```python
from build123d import *

# Parameters (mm, degrees)
SKETCH010_R             = 4
SKETCH010_R_2           = 1.5
PAD_DEPTH               = 10
POCKET003_DEPTH         = 5
POCKET004_DEPTH         = 2.7
PAD010_DEPTH            = 20
FILLET001_R             = 9
FILLET002_R             = 3
FILLET003_R             = 3
FILLET004_R             = 0.9
CHAMFER_SIZE            = 2
FILLET005_R             = 0.9
FILLET006_R             = 1
FILLET007_R             = 0.5
FILLET008_R             = 0.3
FILLET009_R             = 1
BODY001_PLACEMENT_ANGLE = 45


with BuildPart() as part:
    # Sketch010 → Pad (new body)
    with BuildSketch(Plane.XY):
        Polygon((-45.961941, -24.748737), (0, 21.213203), (21.213203, 0), (-24.748737, -45.961941), align=None)
        with Locations((-7.071068, -7.071068)):
            Circle(SKETCH010_R, mode=Mode.SUBTRACT)
        with Locations((-7.071068, 7.071068)):
            Circle(SKETCH010_R_2, mode=Mode.SUBTRACT)
        with Locations((7.071068, -7.071068)):
            Circle(SKETCH010_R_2, mode=Mode.SUBTRACT)
    extrude(amount=PAD_DEPTH)

    # Sketch011 → Pocket003 (cut)
    with BuildSketch(Plane.XY.offset(10)):
        Polygon((-47.335856, -39.41626), (26.386553, 34.306149), (34.306149, 26.386553), (-39.41626, -47.335856), align=None)
    extrude(amount=-POCKET003_DEPTH, mode=Mode.SUBTRACT)

    # Sketch017 → Pocket004 (cut)
    with BuildSketch(Plane.XY.offset(10)):
        with BuildLine():
            ThreePointArc((-5.6, 10.6), (-9.135534, 9.135534), (-10.6, 5.6))
            Line((-10.6, 5.6), (-10.6, -5.6))
            ThreePointArc((-10.6, -5.6), (-9.135534, -9.135534), (-5.6, -10.6))
            Line((-5.6, -10.6), (5.6, -10.6))
            ThreePointArc((5.6, -10.6), (9.135534, -9.135534), (10.6, -5.6))
            Line((10.6, -5.6), (10.6, 5.6))
            ThreePointArc((10.6, 5.6), (9.135534, 9.135534), (5.6, 10.6))
            Line((5.6, 10.6), (-5.6, 10.6))
        make_face()
    extrude(amount=-POCKET004_DEPTH, mode=Mode.SUBTRACT)

    # Sketch023 → Pad010 (join)
    with BuildSketch(Plane.XY.offset(10)):
        Polygon((-41.7193, -21.92031), (-39.59798, -24.041631), (-43.133514, -27.577164), (-45.254834, -25.455844), align=None)
        Polygon((-24.960869, -5.16188), (-22.839549, -7.2832), (-19.304015, -3.747666), (-21.425335, -1.626346), align=None)
    extrude(amount=PAD010_DEPTH)

    # Fillet001
    fillet001_edges = [part.edges().sort_by_distance(p)[0] for p in [
        (0, 21.213203, 5),
        (21.213203, 0, 5),
    ]]
    fillet(fillet001_edges, radius=FILLET001_R)

    # Fillet002
    fillet002_edges = [part.edges().sort_by_distance(p)[0] for p in [
        (-45.961941, -24.748737, 5),
        (-24.748737, -45.961941, 5),
    ]]
    fillet(fillet002_edges, radius=FILLET002_R)

    # Fillet003
    fillet003_edges = [part.edges().sort_by_distance(p)[0] for p in [
        (-41.365747, -25.809398, 10),
        (-21.071782, -5.515433, 10),
        (-40.65864, -22.98097, 10),
        (-20.364675, -2.687006, 10),
        (-23.900209, -6.22254, 10),
    ]]
    fillet(fillet003_edges, radius=FILLET003_R)

    # Fillet004
    fillet004_edges = [part.edges().sort_by_distance(p)[0] for p in [
        (-25.102291, -3.889087, 10),
        (-3.889087, -25.102291, 10),
    ]]
    fillet(fillet004_edges, radius=FILLET004_R)

    # Chamfer
    chamfer_edges = [part.edges().sort_by_distance(p)[0] for p in [
        (5.571068, -7.071068, 0),
        (-8.571068, 7.071068, 0),
    ]]
    chamfer(chamfer_edges, length=CHAMFER_SIZE)

    # Fillet005
    fillet005_edges = [part.edges().sort_by_distance(p)[0] for p in [
        (-40.163665, -30.547013, 10),
    ]]
    fillet(fillet005_edges, radius=FILLET005_R)

    # Fillet006
    fillet006_edges = [part.edges().sort_by_distance(p)[0] for p in [
        (-22.839549, -7.2832, 21.5),
        (-19.304015, -3.747666, 21.5),
    ]]
    fillet(fillet006_edges, radius=FILLET006_R)

    # Fillet007
    fillet007_edges = [part.edges().sort_by_distance(p)[0] for p in [
        (-39.315137, -31.395541, 7.05),
        (-31.395541, -39.315137, 7.05),
    ]]
    fillet(fillet007_edges, radius=FILLET007_R)

    # Fillet008
    fillet008_edges = [part.edges().sort_by_distance(p)[0] for p in [
        (6.646804, 14.5664, 7.05),
        (14.5664, 6.646804, 7.05),
    ]]
    fillet(fillet008_edges, radius=FILLET008_R)

    # Fillet009
    fillet009_edges = [part.edges().sort_by_distance(p)[0] for p in [
        (-25.102291, -3.889087, 0),
    ]]
    fillet(fillet009_edges, radius=FILLET009_R)


with BuildPart() as part_1:
    # Body001 placement: moved
    add(part.part.moved(Location((-4.949747, 51.618795, -12))).rotate(Axis((-4.949747, 51.618795, -12), (0, 0, 1)), BODY001_PLACEMENT_ANGLE))


solid = part_1.part
```
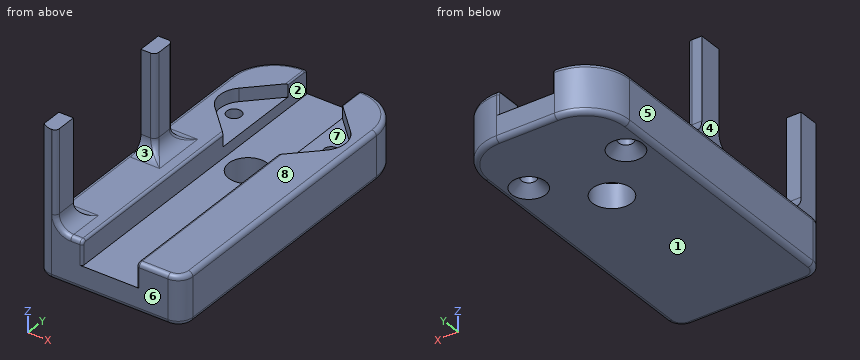
Check sheet for the modelled part. Datum: model origin and axes. Units: mm. Face numbers are marked on the shaded views. A direction names the side the tool comes from. Round coordinates to 2 decimals unless told otherwise and drop trailing zeros. Order: outer loops, then holes, each group sorted by start corner. A loop starts at its lowest first (then second) coordinate and runs counter-clockwise, first axis right, second up. Notation, with made-up numbers: (-31, 47) - (2, 47) arc R22 cw to (2, 74) - close; hole circle Ø2 at (55.25, 58). An arc over 180 degrees is marked (long way). Write item = value, one per line.
Q1. Section check A-A (z = -4). Record the boundary of the cut face in (x, y), and give its area (3 significant figures).
Computed:
outline = (-19.95, 4.62) arc R3 ccw to (-16.95, 1.62) - (-11.05, 1.62) arc R0.5 ccw to (-10.55, 2.12) - (-10.55, 42.23) - (-16.4, 48.08) arc R5 cw to (-16.4, 55.15) - (-10.55, 61.01) - (-10.55, 66.32) arc R0.3 ccw to (-10.85, 66.62) - (-10.95, 66.62) arc R9 ccw to (-19.95, 57.62) - close; (0.65, 2.12) arc R0.5 ccw to (1.15, 1.62) - (7.05, 1.62) arc R3 ccw to (10.05, 4.62) - (10.05, 57.62) arc R9 ccw to (1.05, 66.62) - (0.95, 66.62) arc R0.3 ccw to (0.65, 66.32) - (0.65, 61.01) - (6.51, 55.15) arc R5 cw to (6.51, 48.08) - (0.65, 42.23) - close
area = 1,020 mm^2
Q2. Section check D-D (y = 33). Record the boundary of the cut face in (x, z).
Computed:
outline = (-19.95, -11) arc R1 ccw to (-18.95, -12) - (9.05, -12) arc R1 ccw to (10.05, -11) - (10.05, -2.9) arc R0.9 ccw to (9.15, -2) - (1.15, -2) arc R0.5 ccw to (0.65, -2.5) - (0.65, -7) - (-10.55, -7) - (-10.55, -2.5) arc R0.5 ccw to (-11.05, -2) - (-12.95, -2) arc R3 cw to (-15.95, 1) - (-15.95, 18) - (-18.95, 18) - (-18.95, -2) - (-19.05, -2) arc R0.9 ccw to (-19.95, -2.9) - close
Q3. Section check C-C (x = 0). Record the boundary of the cut face in (y, z), and give its area (3 significant figures).
Computed:
outline = (1.62, -11) arc R1 ccw to (2.62, -12) - (65.62, -12) arc R1 ccw to (66.62, -11) - (66.62, -7) - (1.62, -7) - close
area = 325 mm^2
Q4. Go/stop test with flat-tipped pins: pin 1 (12 mm diameter, centred on y = 14.5, z = 2.5, fed in from -X); pin 2 (6 mm diameter, centred on x = 4.5, y = 54, fed in from +Z); pin 3 (1 mm diameter, centred on x = -12.5, y = 50, fed in from -Z); pin 4 (6 mm diameter, centred on x = -13, y = 49.5, fed in from +Z). Record where each tip stops, or that it passes through.
Computed:
pin_1 = -19.95
pin_2 = -2
pin_3 = -11.94
pin_4 = -4.7
Q5. Thickness scan on line 1 along X through (y, z) = (25, -6.5); line 2 along Z through (x, y) = (4, 59); line 3 along Z through (x, y) = (-6, 35). Record the ranges inside material, lowest first.
Computed:
line_1 = -19.95 to -10.55, 0.65 to 10.05
line_2 = -12 to -2
line_3 = -12 to -7
Q6. Draft check along Z on the marked faces 1, 2 and 3. Enter one of: pulls with the +Z half, pulls with the -Z half, needs draft (parallel to the pull), parting line crosses it, or undercut.
Computed:
face_1 = pulls with the -Z half
face_2 = needs draft
face_3 = pulls with the +Z half
Q7. Tool access check on the marked faces 4, 5, 6, 7 and 8. Record the directions out of +Z, -Z, +X, -X, +Y, -Y that give a thin tool (end or side, any length) a straight path to the whole face; none if there is none.
Computed:
face_4 = +Z, -X, +Y, -Y
face_5 = +Z, -Z, -X, +Y, -Y
face_6 = +Z, -Z, +X, -X, -Y
face_7 = +Z
face_8 = +Z, +X, +Y, -Y
Q8. Section check B-B (y = 41.5). Record the boundary of the cut face in (x, z).
Computed:
outline = (-19.95, -11) arc R1 ccw to (-18.95, -12) - (-8.95, -12) - (-8.95, -7) - (-10.55, -7) - (-10.55, -2.5) arc R0.5 ccw to (-11.05, -2) - (-19.05, -2) arc R0.9 ccw to (-19.95, -2.9) - close; (-0.95, -12) - (9.05, -12) arc R1 ccw to (10.05, -11) - (10.05, -2.9) arc R0.9 ccw to (9.15, -2) - (1.15, -2) arc R0.5 ccw to (0.65, -2.5) - (0.65, -7) - (-0.95, -7) - close
